from build123d import *

# Parameters (mm, degrees)
SKICA1_R                 = 12.5
P_IDAT_VYSUNUT_M1_DEPTH  = 48
SKICA2_R                 = 3.5
P_IDAT_VYSUNUT_M2_DEPTH  = 2.5
SKICA3_R                 = 2
P_IDAT_VYSUNUT_M3_DEPTH  = 10
SKICA4_W                 = 4
SKICA4_H                 = 1.5
P_IDAT_VYSUNUT_M4_DEPTH  = 4
SKICA5_R                 = 1.65
ODEBRAT_VYSUNUT_M1_DEPTH = 4


with BuildPart() as part:
    # Skica1 → Přidat vysunutím1 (new body)
    with BuildSketch(Plane.XY):
        Circle(SKICA1_R)
    extrude(amount=P_IDAT_VYSUNUT_M1_DEPTH)

    # Skica2 → Přidat vysunutím2 (add)
    with BuildSketch(Plane.XY.offset(48)):
        Circle(SKICA2_R)
    extrude(amount=P_IDAT_VYSUNUT_M2_DEPTH)

    # Skica3 → Přidat vysunutím3 (add)
    with BuildSketch(Plane.XY.offset(50.5)):
        Circle(SKICA3_R)
    extrude(amount=P_IDAT_VYSUNUT_M3_DEPTH)

    # Skica4 → Přidat vysunutím4 (add)
    with BuildSketch(Plane(origin=(0, 0, 0), x_dir=(-1, 0, 0), z_dir=(0, 0, -1))):
        with Locations((-6.5, 0.25)):
            Rectangle(SKICA4_W, SKICA4_H)
        with Locations((6.5, 0.25)):
            Rectangle(SKICA4_W, SKICA4_H)
    extrude(amount=P_IDAT_VYSUNUT_M4_DEPTH)

    # Skica5 → Odebrat vysunutím1 (cut)
    with BuildSketch(Plane.XY.offset(48)):
        with Locations((0, 8.5)):
            Circle(SKICA5_R)
        with Locations((0, -8.5)):
            Circle(SKICA5_R)
    extrude(amount=-ODEBRAT_VYSUNUT_M1_DEPTH, mode=Mode.SUBTRACT)


solid = part.part
Here's how the part is built. I have some questions about the finished solid (model axes, mm). A direction names the side the tool comes from. Round coordinates to 2 decimals unless told otherwise and drop trailing zeros. Write each loop counter-clockwise with the first axis right and the second up, starting at its lowest first coordinate (ties: lowest second). Pieces come first, ordered by that corner, then holes.
1. Suppose I cut it at D-D (x = -7.5). List the corners of the cut face in (y, z) for me.
2. Suppose I cut it at C-C (z = 38). List the corners of the cut face in (x, y) for me.
3. If we mould it in two halves opening along Y, with no side actions, what happens to faces 1 (the flat face through (7, -0.5, -2)), 2 (the cylindrical face through (-0.215, -6.864, 46.028)), 3 (the flat face through (0, -8, 44)), 4 (the flat face through (0, 0, 0))? For each: released by +Y, released by -Y, zero draft, split by the parting line, or undercut.
4. I need wall thicknesses on L1, parallel to Y at x = 0, z = 45.2; L2, parallel to Z at x = 8.25, y = 9; L3, parallel to Z at x = 0.5, y = -2. Which ranges of each line are inside material? Lowest first, please.
5. For faces 5 (the flat face through (0, 9, 44)), 6 (the flat face through (4.5, 0, -2)), 7 (the flat face through (-8.5, 0, -2)), which set-ups out of +Z, -Z, +X, -X, +Y, -Y let a thin tool reach every point of the face, with its end or its side?
6. Will these pins go through, and if not, where does the flat tip stop? pin 1 Ø2 at (x, y) = (9.5, -5.5) entering from +Z; pin 2 Ø6 at (y, z) = (7, 19) entering from -X; pin 3 Ø3 at (x, z) = (5.5, -1) entering from +Y.
7. Suppose I cut it at A-A (x = 0). List the corners of the cut face in (y, z) for me, and give its area (3 significant figures).
8. Suppose I cut it at B-B (y = -2.75). List the corners of the cut face in (x, z) for me.
Answer sheet:
1. outline: (-10, 0) - (-0.5, 0) - (-0.5, -4) - (1, -4) - (1, 0) - (10, 0) - (10, 48) - (-10, 48) - close
2. outline: circle Ø25 at (0, 0)
3. face 1: released by -Y
3. face 2: undercut
3. face 3: undercut
3. face 4: zero draft
4. L1: y = -12.5 to -10.15, -6.85 to 6.85, 10.15 to 12.5
4. L2: z = 0 to 48
4. L3: z = 0 to 50.5
5. face 5: +Z
5. face 6: -Z, +Y, -Y
5. face 7: -Z, -X, +Y, -Y
6. pin 1: stops at z = 48
6. pin 2: stops at x = -11.84
6. pin 3: stops at y = 11.71
7. outline: (-12.5, 0) - (12.5, 0) - (12.5, 48) - (10.15, 48) - (10.15, 44) - (6.85, 44) - (6.85, 48) - (3.5, 48) - (3.5, 50.5) - (2, 50.5) - (2, 60.5) - (-2, 60.5) - (-2, 50.5) - (-3.5, 50.5) - (-3.5, 48) - (-6.85, 48) - (-6.85, 44) - (-10.15, 44) - (-10.15, 48) - (-12.5, 48) - close
7. area: 1,230 mm2
8. outline: (-12.19, 0) - (12.19, 0) - (12.19, 48) - (2.17, 48) - (2.17, 50.5) - (-2.17, 50.5) - (-2.17, 48) - (-12.19, 48) - close
